The model under review builds one solid part; all positions refer to its coordinate system, in mm. A direction names the side the tool comes from. Give positions to 0.01 mm unless a question says otherwise; leave off trailing zeros. Order: outer loops, then holes, each group sorted by start corner. A loop starts at its lowest first (then second) coordinate and runs counter-clockwise, first axis right, second up. Notation, with made-up numbers: M 62.25,62.25 L 112.25,62.25 A26 ccw 112.25,81.25 Z; hole C -5.5,-24 d2. An arc over 180 degrees is marked long. One line per question, with ' | ' between items. Start each with the question number.
1. We need section A-A on x = 0. Write out the cut boundary in (y, z), then the cut area to 3 significant figures.
2. The part is to be moulded in two halves that separate along Z. For faces 1 (the face through (-82, 0, 46)), 2 (the face through (84.932, 15.605, 1.041)), 3 (the face through (-51.277, 2.028, 84.494)), 4 (the face through (47.465, 2.028, -86.493)), say which applies: +Z half, -Z half, draft (parallel to the pull), parting line (faces both ways), or undercut.
3. Wall thickness on L1, parallel to Y at x = 52, z = 41.5; L2, parallel to X at y = 3.75, z = 21; L3, parallel to Y at x = -20.5, z = -95: over which ranges is each line inside the solid? List them lowest first.
4. Insertion check: P1, Ø12, axis at x = -42.5, y = 6, coming from the -Z side; P2, Ø6, axis at x = 77, y = 15, coming from the +Z side; P3, Ø8, axis at x = -6, y = 10.5, coming from the +Z side; P4, Ø10, axis at y = 15, z = 31, coming from the -X side. Each pin has a flat end and moves straight along its axis. Give the tip position at first contact, or say it passes through.
5. For faces 5 (the face through (83, 0, 46)), 6 (the face through (-1, 4, 8)), 7 (the face through (-0.658, 2.028, -92.498)), 8 (the face through (-47.535, 2.028, -86.654)), list the 3-axis set-ups (+Z, -Z, +X, -X, +Y, -Y) from which the entire face can be reached by the end or side of a thin tool; tool diameter is ignored.
6. We need section B-B on z = 68. Write out the cut boundary in (x, y).
7. We need section C-C on y = 12.25. Write out the cut boundary in (x, z).
8. We need section D-D on x = -66. Write out the cut boundary in (y, z), then the cut area to 3 significant figures.
```python
from build123d import *
from build123d.topology import SkipClean

# Parameters (mm, degrees)
SKETCH1_W           = 105
SKETCH1_H           = 8
CUT_EXTRUDE1_START  = -4
CUT_EXTRUDE1_DEPTH  = 4
BOSS_EXTRUDE1_DEPTH = 4
BOSS_EXTRUDE2_DEPTH = 4
SKETCH5_W           = 8
SKETCH5_H           = 15


with BuildPart() as part:
    # Sketch1 → Revolve1 (revolve)
    with BuildSketch(Plane.XY):
        with Locations((52.5, 4)):
            Rectangle(SKETCH1_W, SKETCH1_H)
    revolve(axis=Axis((0, 8, 0), (0, -1, 0)))

    # Sketch2 → Cut-Extrude1 (cut)
    with BuildSketch(Plane.XZ.offset(CUT_EXTRUDE1_START)):
        with BuildLine():
            Line((47.488838396, 79.379217858), (54.960927959, 89.466733471))
            ThreePointArc((54.960927959, 89.466733471), (-90.932667397, -52.5), (104.960927959, 2.864193092))
            Line((104.960927959, 2.864193092), (92.488838396, 1.436931518))
            ThreePointArc((92.488838396, 1.436931518), (80.10734985, 46.25), (47.488838396, 79.379217858))
        make_face()
    extrude(amount=CUT_EXTRUDE1_DEPTH, mode=Mode.SUBTRACT)

    # Sketch3 → Boss-Extrude1 (add)
    with SkipClean():  # the faces are left unmerged after this step: merging them gives an invalid solid
        with BuildSketch(Plane.XZ.offset(-4)):
            with BuildLine():
                Line((-92.488838396, 1.436931518), (-104.960927959, 2.864193092))
                ThreePointArc((-104.960927959, 2.864193092), (-90.932667397, 52.5), (-54.960927959, 89.466733471))
                Line((-54.960927959, 89.466733471), (-47.488838396, 79.379217858))
                ThreePointArc((-47.488838396, 79.379217858), (-80.10734985, 46.25), (-92.488838396, 1.436931518))
            make_face()
        extrude(amount=BOSS_EXTRUDE1_DEPTH)

    # Sketch4 → Boss-Extrude2 (add)
    with SkipClean():  # the faces are left unmerged after this step: merging them gives an invalid solid
        with BuildSketch(Plane.XZ.offset(-4)):
            with BuildLine():
                Line((-50, -92.330926563), (-45, -80.816149376))
                ThreePointArc((-45, -80.816149376), (0, -92.5), (45, -80.816149376))
                Line((45, -80.816149376), (50, -92.330926563))
                ThreePointArc((50, -92.330926563), (0, -105), (-50, -92.330926563))
            make_face()
        extrude(amount=BOSS_EXTRUDE2_DEPTH)

    # Sketch5 → Revolve2 (revolve)
    with SkipClean():  # the faces are left unmerged after this step: merging them gives an invalid solid
        with BuildSketch(Plane.XY, mode=Mode.PRIVATE) as revolve2_sk:
            with Locations((81, 15.5)):
                Rectangle(SKETCH5_W, SKETCH5_H)
        revolve(revolve2_sk.sketch.rotate(Axis((77, 23, 0), (0, -1, 0)), 270), axis=Axis((77, 23, 0), (0, -1, 0)))


solid = part.part
```
Entries:
1) outline: M 0,-105 L 8,-105 L 8,105 L 4,105 L 4,-92.5 L 0,-92.5 Z | area: 890 mm^2
2) face 1: draft | face 2: parting line | face 3: +Z half | face 4: undercut
3) L1: y = 4 to 8 | L2: x = -102.88 to -90.08, 90.08 to 102.88 | L3: y = 0 to 8
4) P1: stops at z = -98.45 | P2: stops at z = 8 | P3: stops at z = 104.96 | P4: passes through
5) face 5: +Z, -Z, +X, -X, -Y | face 6: -Y | face 7: +Z, -Y | face 8: -X, -Y
6) outline: M -80.01,0 L -62.71,0 L -62.71,4 L 62.71,4 L 62.71,0 L 80.01,0 L 80.01,8 L -80.01,8 Z
7) outline: C 77,0 d16
8) outline: M 0,64.81 L 4,64.81 L 4,-81.66 L 8,-81.66 L 8,81.66 L 0,81.66 Z | area: 721 mm^2
